Print and shaded views of the part. All mm, measured from the part's lowest x, y and z. A direction names the side the tool comes from. Give positions to 0.01 mm unless a question says otherwise; leave off trailing zeros. Loops run counter-clockwise (first coordinate to the right, second up) from the corner with the lowest first, then second, coordinate; pieces in that order, holes last.
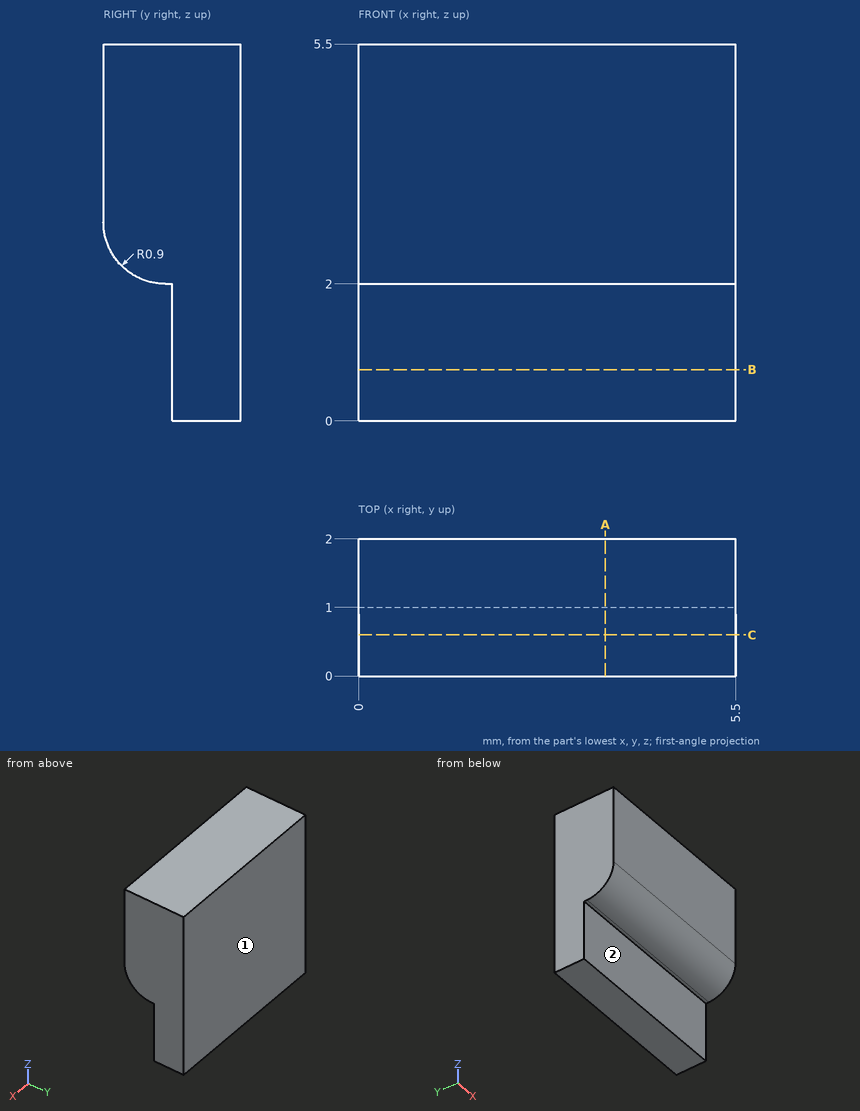
1. Tool access for the marked faces 1 and 2: list every direction of +Z, -Z, +X, -X, +Y, -Y with a clear straight run to the whole face (end or side of a thin tool).
Responses:
face 1: +Z, -Z, +X, -X, +Y
face 2: -Z, +X, -X, -Y
2. Probe line 1 along Y through (x, z) = (1.5, 0.65); line 2 along Z through (x, y) = (0.95, 0.55); line 3 along Z through (x, y) = (0.65, 0.4). List the from-to ranges inside material, lowest first.
Responses:
line 1: y = 1 to 2
line 2: z = 2.07 to 5.5
line 3: z = 2.15 to 5.5
3. Saw through at C-C, the plane y = 0.6. List the corners of the cut face in (x, z).
Responses:
outline: (0, 2.05) - (5.5, 2.05) - (5.5, 5.5) - (0, 5.5) - close
4. Saw through at B-B, the plane z = 0.75. List the corners of the cut face in (x, y), and give its area (3 significant figures).
Responses:
outline: (0, 1) - (5.5, 1) - (5.5, 2) - (0, 2) - close
area: 5.50 mm2
5. Saw through at A-A, the plane x = 3.6. List the corners of the cut face in (y, z), and give its area (3 significant figures).
Responses:
outline: (0, 2.9) arc R0.9 ccw to (0.9, 2) - (1, 2) - (1, 0) - (2, 0) - (2, 5.5) - (0, 5.5) - close
area: 8.83 mm2
